```python
from build123d import *

# Parameters (mm, degrees)
F1_DEPTH = 292
F3_R     = 12
F2_R     = 12.973192
F2_R_2   = 12.9794


with BuildPart() as f1:
    # F0 (on Top) → F1 (new body)
    with BuildSketch(Plane.XY):
        with BuildLine():
            Line((20.542224, -6.856897), (0, 0))
            Line((0, 0), (-125, 0))
            Line((-125, 0), (-125, -8))
            Line((-125, -8), (0, -8))
            Line((0, -8), (17.58743, -14.299388))
            ThreePointArc((17.58743, -14.299388), (39.685209, 18.77169), (4.619105, 0))
            Line((4.619105, 0), (13.043561, 0))
            ThreePointArc((13.043561, 0), (32.935269, 14.224762), (20.542224, -6.856897))
        make_face()
    extrude(amount=F1_DEPTH)

    # F3 (on Front) → F4 section 0
    with BuildSketch(Plane.XZ):
        with Locations((-54.026808, 249.026808)):
            Circle(F3_R)
    # F2 (on face) → F4 section 1
    with BuildSketch(Plane.XZ.offset(8)):
        with Locations((-54.026808, 249.026808)):
            Circle(F2_R)
    loft(mode=Mode.SUBTRACT)

    # F2 (on face) → F5 section 0
    with BuildSketch(Plane.XZ.offset(8)):
        with Locations((-77.376664, 146)):
            Circle(F2_R_2)
    # F3 (on Front) → F5 section 1
    with BuildSketch(Plane.XZ):
        with Locations((-77.376664, 146)):
            Circle(F3_R)
    loft(mode=Mode.SUBTRACT)


solid = f1.part
```
Could you check a few things on this model? Use its own coordinates, in mm. A direction names the side the tool comes from. Coordinates: 2 decimals unless noted, no trailing zeros. Loops run counter-clockwise (first coordinate to the right, second up) from the corner with the lowest first, then second, coordinate; pieces in that order, holes last. Notation, with made-up numbers: M -18.5,49 L 19.5,49 A22 ccw 19.5,72 Z; hole C 53.5,17 d3. An arc over 180 degrees is marked long. Put each result on its own line as item: value. Start each with the question number.
(1) Suppose I cut it at C-C on z = 93. Please give me the cut outline in (x, y), then the cut area to 3 significant figures.
(2) Suppose I cut it at A-A on x = 24.5. Please give me the cut outline in (y, z), then the cut area to 3 significant figures.
(3) Will these pins go through, and if not, where does the flat tip stop? P1, Ø8, axis at x = -43, z = 137, coming from the -Y side; P2, Ø6, axis at x = -35, z = 42, coming from the +Y side; P3, Ø6.5, axis at x = 8.5, z = 202, coming from the -Y side.
(4) Suppose I cut it at B-B on y = 5. Please give me the cut outline in (x, z), then the cut area to 3 significant figures.
(5) Thinking about a two-plate mould opening in Z: for faces 1 (the face through (40.186, 18.199, 143.956)), 2 (the face through (-78.97, -2.17, 158.16)), 3 (the face through (-22, -2, 292)), which applies, pulls with the +Z half, pulls with the -Z half, needs draft (parallel to the pull), parting line crosses it, or undercut?
(6) For faces 4 (the face through (-63, -8, 144)), 5 (the face through (-62, 0, 144)), 6 (the face through (9, 0, 144)), which set-ups out of +Z, -Z, +X, -X, +Y, -Y let a thin tool reach every point of the face, with its end or its side?
(7) Suppose I cut it at D-D on x = -31.5. Please give me the cut outline in (y, z), then the cut area to 3 significant figures.
(8) I need wall thicknesses on line 1 (X direction, y = 5, z = 70); line 2 (Y direction, x = 24.5, z = 110.5); line 3 (Y direction, x = -115, z = 139.5). Which ranges of each line are inside material? Lowest first, please. Write a range as from..to.
Solutions:
1. outline: M -125,-8 L 0,-8 L 17.59,-14.3 A20.5 ccw long 4.62,0 L 13.04,0 A12.5 cw long 20.54,-6.86 L 0,0 L -125,0 Z
1. area: 1,860 mm2
2. outline: M -15.5,0 L -7.5,0 L -7.5,292 L -15.5,292 Z; M 17.5,0 L 25.5,0 L 25.5,292 L 17.5,292 Z
2. area: 4,670 mm2
3. P1: stops at y = -8
3. P2: stops at y = 0
3. P3: stops at y = -12.21
4. outline: M 4,0 L 12,0 L 12,292 L 4,292 Z; M 37,0 L 45,0 L 45,292 L 37,292 Z
4. area: 4,670 mm2
5. face 1: needs draft
5. face 2: undercut
5. face 3: pulls with the +Z half
6. face 4: +Z, -Z, -X, -Y
6. face 5: +Z, -Z, -X, +Y
6. face 6: +Z, -Z
7. outline: M -8,0 L 0,0 L 0,292 L -8,292 Z
7. area: 2,340 mm2
8. line 1: x = 4..12, 37..45
8. line 2: y = -15.5..-7.5, 17.5..25.5
8. line 3: y = -8..0
